Read the model definition and answer for the solid it produces. Units are mm, in the model's axes. Give positions to 0.01 mm unless a question says otherwise; leave off trailing zeros. Write each loop counter-clockwise with the first axis right and the second up, starting at its lowest first coordinate (ties: lowest second). Pieces come first, ordered by that corner, then holes. Notation, with made-up numbers: (46.5, 11.25) - (77.5, 11.25) arc R21 ccw to (77.5, 29.25) - close; hole circle Ø5 at (70, 69.5). An arc over 180 degrees is marked (long way). Use CSV: the item, a comma, the result in double quotes. Start each with the question number.
from build123d import *

# Parameters (mm, degrees)
F0_R     = 10
F0_R_2   = 1
F1_DEPTH = 40


with BuildPart() as f1:
    # F0 (on Front) → F1 (new body)
    with BuildSketch(Plane.XZ):
        Circle(F0_R)
        with BuildLine():
            ThreePointArc((6.6435448727, 4.4568275179), (7.0165111824, 3.8429898293), (7.3329177707, 3.1981740052))
            ThreePointArc((7.3329177707, 3.1981740052), (8.5333245383, 2.0924606947), (8.9772542605, 0.5219497159))
            ThreePointArc((8.9772542605, 0.5219497159), (8.6602558801, -0.8202508315), (7.776252721, -1.8788011123))
            ThreePointArc((7.776252721, -1.8788011123), (6.8566594958, -4.1214342842), (5.3076404374, -5.9857291107))
            ThreePointArc((5.3076404374, -5.9857291107), (3.5152152369, -8.2851229223), (0.6161482026, -7.9762372954))
            ThreePointArc((0.6161482026, -7.9762372954), (-1.8008926237, -7.7946639285), (-4.0526155804, -6.8975580431))
            ThreePointArc((-4.0526155804, -6.8975580431), (-6.7933588965, -5.9034121407), (-7.3954521896, -3.0507846385))
            ThreePointArc((-7.3954521896, -3.0507846385), (-7.630756176, -2.4024071642), (-7.8093348718, -1.7361707463))
            ThreePointArc((-7.8093348718, -1.7361707463), (-8.9605366896, -0.8418920566), (-7.9960562334, 0.251166702))
            ThreePointArc((-7.9960562334, 0.251166702), (-7.9383510901, 0.9912527276), (-7.8122946094, 1.7228038007))
            ThreePointArc((-7.8122946094, 1.7228038007), (-7.7137419327, 4.6366135697), (-5.186789018, 6.0907486964))
            ThreePointArc((-5.186789018, 6.0907486964), (-3.1246357662, 7.3645537087), (-0.7756480184, 7.9623093479))
            ThreePointArc((-0.7756480184, 7.9623093479), (2.0260042016, 8.7689969195), (4.189840284, 6.8150743499))
            ThreePointArc((4.189840284, 6.8150743499), (4.7806533049, 6.4144644343), (5.3334042334, 5.9627845243))
            ThreePointArc((5.3334042334, 5.9627845243), (6.4214881928, 6.1733853396), (7.035627896, 5.2508281158))
            ThreePointArc((7.035627896, 5.2508281158), (6.9322652186, 4.8080623632), (6.6435448727, 4.4568275179))
        make_face(mode=Mode.SUBTRACT)
        with BuildLine():
            ThreePointArc((-2.5712473173, 1.5455378459), (-1.1717384371, 2.7617076302), (0.6753346935, 2.9229989825))
            ThreePointArc((0.6753346935, 2.9229989825), (-0.9731935316, 3.9487207499), (-1.6483458018, 5.7691382474))
            ThreePointArc((-1.6483458018, 5.7691382474), (-2.3434768246, 5.5234152815), (-3.0032221992, 5.1942907526))
            ThreePointArc((-3.0032221992, 5.1942907526), (-2.3660024763, 4.2273377279), (-2.1424946218, 3.0910757132))
            ThreePointArc((-2.1424946218, 3.0910757132), (-2.2516693146, 2.2891224456), (-2.5712473173, 1.5455378459))
        make_face()
        with BuildLine():
            ThreePointArc((0.6753346935, 2.9229989825), (2.2644529469, 1.9678040683), (2.9886271289, 0.2609748731))
            ThreePointArc((2.9886271289, 0.2609748731), (3.454723253, 2.1457838566), (4.9774096583, 3.3504317772))
            ThreePointArc((4.9774096583, 3.3504317772), (4.528905931, 3.9356080938), (4.0120173703, 4.4613581587))
            ThreePointArc((4.0120173703, 4.4613581587), (2.6067344642, 3.1216079734), (0.6753346935, 2.9229989825))
        make_face()
        with BuildLine():
            ThreePointArc((2.9886271289, 0.2609748731), (2.9971554336, 0.1306112807), (3, 0))
            ThreePointArc((3, 0), (2.5015210631, -1.6560170201), (1.1717384193, -2.7617076378))
            ThreePointArc((1.1717384193, -2.7617076378), (3.1083299118, -2.6225533829), (4.7245541465, -3.6984575321))
            ThreePointArc((4.7245541465, -3.6984575321), (5.1424946218, -3.0910757132), (5.4827852975, -2.4370197745))
            ThreePointArc((5.4827852975, -2.4370197745), (3.7743508626, -1.5145218945), (2.9886271289, 0.2609748731))
        make_face()
        with BuildLine():
            ThreePointArc((-0.5795221486, -4.8480805477), (0.0456612251, -3.5946738602), (1.1717384193, -2.7617076378))
            ThreePointArc((1.1717384193, -2.7617076378), (-0.675334733, -2.9229989734), (-2.2644529693, -1.9678040425))
            ThreePointArc((-2.2644529693, -1.9678040425), (-1.7188028292, -2.8852174249), (-1.528905931, -3.9356080938))
            ThreePointArc((-1.528905931, -3.9356080938), (-1.5482183493, -4.2754632692), (-1.6059069578, -4.6109428277))
            Line((-1.6059069578, -4.6109428277), (-0.5795221486, -4.8480805477))
        make_face()
        with BuildLine():
            ThreePointArc((-0.6234697034, -5.9675192106), (-0.654213992, -5.4057302436), (-0.5795221486, -4.8480805477))
            Line((-0.5795221486, -4.8480805477), (-1.6059069578, -4.6109428277))
            ThreePointArc((-1.6059069578, -4.6109428277), (-1.783407838, -5.1448393461), (-2.057474614, -5.636204238))
            ThreePointArc((-2.057474614, -5.636204238), (-1.3506694677, -5.8459979464), (-0.6234697034, -5.9675192106))
        make_face()
        with BuildLine():
            ThreePointArc((0.6161482026, -7.9762372954), (-0.2095198229, -7.0989177785), (-0.6234697034, -5.9675192106))
            ThreePointArc((-0.6234697034, -5.9675192106), (-1.3506694677, -5.8459979464), (-2.057474614, -5.636204238))
            ThreePointArc((-2.057474614, -5.636204238), (-2.9257780157, -6.4713487918), (-4.0526155804, -6.8975580431))
            ThreePointArc((-4.0526155804, -6.8975580431), (-1.8008926237, -7.7946639285), (0.6161482026, -7.9762372954))
        make_face()
        with BuildLine():
            ThreePointArc((-5.8681107652, -1.2511099262), (-3.9437276347, -0.993233821), (-2.2644529693, -1.9678040425))
            ThreePointArc((-2.2644529693, -1.9678040425), (-2.9886271299, -0.2609748613), (-2.5712473173, 1.5455378459))
            ThreePointArc((-2.5712473173, 1.5455378459), (-4.0561899268, 0.2946597731), (-5.996143389, 0.2150917455))
            ThreePointArc((-5.996143389, 0.2150917455), (-5.9772542605, -0.5219497159), (-5.8681107652, -1.2511099262))
        make_face()
        with BuildLine():
            ThreePointArc((-7.3954521896, -3.0507846385), (-6.8162171978, -1.9944210424), (-5.8681107652, -1.2511099262))
            ThreePointArc((-5.8681107652, -1.2511099262), (-5.9772542605, -0.5219497159), (-5.996143389, 0.2150917455))
            ThreePointArc((-5.996143389, 0.2150917455), (-7.0587335663, 0.7828234939), (-7.8122946094, 1.7228038007))
            ThreePointArc((-7.8122946094, 1.7228038007), (-7.9383510901, 0.9912527276), (-7.9960562334, 0.251166702))
            ThreePointArc((-7.9960562334, 0.251166702), (-7.2689095521, -0.0303182964), (-6.9649215018, -0.7483484948))
            ThreePointArc((-6.9649215018, -0.7483484948), (-7.2047943315, -1.3981228287), (-7.8093348718, -1.7361707463))
            ThreePointArc((-7.8093348718, -1.7361707463), (-7.630756176, -2.4024071642), (-7.3954521896, -3.0507846385))
        make_face()
        with BuildLine():
            ThreePointArc((7.776252721, -1.8788011123), (6.686726826, -2.3929514281), (5.4827852975, -2.4370197745))
            ThreePointArc((5.4827852975, -2.4370197745), (5.1424946218, -3.0910757132), (4.7245541465, -3.6984575321))
            ThreePointArc((4.7245541465, -3.6984575321), (5.1845357791, -4.5598884178), (5.3434768246, -5.5234152815))
            ThreePointArc((5.3434768246, -5.5234152815), (5.3345043101, -5.755265623), (5.3076404374, -5.9857291107))
            ThreePointArc((5.3076404374, -5.9857291107), (6.8566594958, -4.1214342842), (7.776252721, -1.8788011123))
        make_face()
        with BuildLine():
            ThreePointArc((4.0120173703, 4.4613581587), (4.528905931, 3.9356080938), (4.9774096583, 3.3504317772))
            ThreePointArc((4.9774096583, 3.3504317772), (6.1707675187, 3.51570198), (7.3329177707, 3.1981740052))
            ThreePointArc((7.3329177707, 3.1981740052), (7.0165111824, 3.8429898293), (6.6435448727, 4.4568275179))
            ThreePointArc((6.6435448727, 4.4568275179), (5.281174409, 4.5944746013), (5.3334042334, 5.9627845243))
            ThreePointArc((5.3334042334, 5.9627845243), (4.7806533049, 6.4144644343), (4.189840284, 6.8150743499))
            ThreePointArc((4.189840284, 6.8150743499), (4.3101890613, 6.3371636776), (4.3506694677, 5.8459979464))
            ThreePointArc((4.3506694677, 5.8459979464), (4.2647768532, 5.1332720901), (4.0120173703, 4.4613581587))
        make_face()
        with BuildLine():
            ThreePointArc((1.1717384193, -2.7617076378), (2.5015210631, -1.6560170201), (3, 0))
            ThreePointArc((3, 0), (2.9971554336, 0.1306112807), (2.9886271289, 0.2609748731))
            ThreePointArc((2.9886271289, 0.2609748731), (2.2644529469, 1.9678040683), (0.6753346935, 2.9229989825))
            ThreePointArc((0.6753346935, 2.9229989825), (-1.1717384371, 2.7617076302), (-2.5712473173, 1.5455378459))
            ThreePointArc((-2.5712473173, 1.5455378459), (-2.9886271299, -0.2609748613), (-2.2644529693, -1.9678040425))
            ThreePointArc((-2.2644529693, -1.9678040425), (-0.675334733, -2.9229989734), (1.1717384193, -2.7617076378))
        make_face()
        Circle(F0_R_2, mode=Mode.SUBTRACT)
        with BuildLine():
            ThreePointArc((-3.0032221992, 5.1942907526), (-2.3434768246, 5.5234152815), (-1.6483458018, 5.7691382474))
            ThreePointArc((-1.6483458018, 5.7691382474), (-1.4367592458, 6.9551603182), (-0.7756480184, 7.9623093479))
            ThreePointArc((-0.7756480184, 7.9623093479), (-3.1246357662, 7.3645537087), (-5.186789018, 6.0907486964))
            ThreePointArc((-5.186789018, 6.0907486964), (-4.0031340801, 5.8662977864), (-3.0032221992, 5.1942907526))
        make_face()
    extrude(amount=F1_DEPTH)


solid = f1.part
(1) The part is cut by section A-A on z = 7.5. Write down the section's boundary in (x, y).
(2) The part is cut by section C-C on y = -24. Give the number of separate pieces and of enclosed holes in the cut face, plus the area to 3 significant figures.
(3) The part is cut by section B-B on x = 0. Write down the section's boundary in (y, z), plus the area to 3 significant figures.
(4) For a pull along Z with two mould halves and no side action, classify faces 1 (the face through (2, 0, 0)), 2 (the face through (0, -20, -1)), 3 (the face through (-2.17, -19.72, -9.76)) as pulls with the +Z half, pulls with the -Z half, needs draft (parallel to the pull), parting line crosses it, or undercut.
(5) Consider probe 1 along Z at (x, y) = (0, -27); probe 2 along Z at (x, y) = (-4.25, -16); probe 3 along Z at (x, y) = (-6, -7). Determine where each line is inside the solid, lowest interval first.
(6) Given P1, Ø2, axis at y = -10.5, z = -8, coming from the +X side; P2, Ø5, axis at x = 8, y = -5.5, coming from the +Z side; P3, Ø1, axis at x = -2, y = -16, coming from the -Z side, each flat-ended and moving along its own axis, determine where each tip first touches the part or whether it passes through.
Reported:
1,outline,"(-6.61, -40) - (-1.15, -40) - (-1.15, 0) - (-6.61, 0) - close; (3.85, -40) - (6.61, -40) - (6.61, 0) - (3.85, 0) - close"
2,separate pieces,"1"
2,enclosed holes,"8"
2,area,"163 mm²"
3,outline,"(-40, -10) - (0, -10) - (0, -7.4) - (-40, -7.4) - close; (-40, -3.65) - (0, -3.65) - (0, -1) - (-40, -1) - close; (-40, 1) - (0, 1) - (0, 3.17) - (-40, 3.17) - close; (-40, 8.52) - (0, 8.52) - (0, 10) - (-40, 10) - close"
3,area,"356 mm²"
4,face 1,"needs draft"
4,face 2,"undercut"
4,face 3,"parting line crosses it"
5,probe 1,"-10 to -7.4, -3.65 to -1, 1 to 3.17, 8.52 to 10"
5,probe 2,"-9.05 to -6.92, -0.95 to 0.23, 5.96 to 9.05"
5,probe 3,"-8 to -6.55, -1.32 to 0.22, 5.97 to 8"
6,P1,"x = 7.14"
6,P2,"z = 8.35"
6,P3,"z = -9.89"
